Can you work these out from the model? Positions are in its coordinate system, mm. A direction names the side the tool comes from. Round coordinates to 2 decimals unless told otherwise and drop trailing zeros. Order: outer loops, then holes, each group sorted by start corner. A loop starts at its lowest first (then second) coordinate and runs counter-clockwise, first axis right, second up. Notation, with made-up numbers: (-10.5, 83.25) - (42.5, 83.25) arc R23 cw to (42.5, 100.25) - close; hole circle Ø7 at (-37.75, 9). An arc over 180 degrees is marked (long way). Write item = value, one per line.
from build123d import *

# Parameters (mm, degrees)
SKETCH1_R              = 5.207
BOSS_EXTRUDE1_DEPTH    = 3.175
SKETCH2_W              = 65.278
SKETCH2_H              = 25.4
BOSS_EXTRUDE2_DEPTH    = 3.175
FILLET1_R              = 3.175
CONVERT_SOLID1_DEPTH   = 65.278
CONVERT_SOLID1_2_DEPTH = 65.278


# Read off the part's stored shape, not the designer's step: Convert-Solid1
with BuildPart() as part:
    # Sketch1 → Boss-Extrude1 (new body)
    with BuildSketch(Plane.XY):
        with BuildLine():
            Line((0, 0), (65.278, 0))
            Line((65.278, 0), (65.278, 66.802))
            ThreePointArc((65.278, 66.802), (56.515, 75.565), (47.752, 66.802))
            ThreePointArc((47.752, 66.802), (32.639, 51.689), (17.526, 66.802))
            ThreePointArc((17.526, 66.802), (8.763, 75.565), (0, 66.802))
            Line((0, 66.802), (0, 0))
        make_face()
        with Locations((8.763, 66.802)):
            Circle(SKETCH1_R, mode=Mode.SUBTRACT)
        with Locations((56.515, 66.802)):
            Circle(SKETCH1_R, mode=Mode.SUBTRACT)
    extrude(amount=BOSS_EXTRUDE1_DEPTH)

    # Sketch2 → Boss-Extrude2 (add)
    with BuildSketch(Plane(origin=(0, 0, 0), x_dir=(1, 0, 0), z_dir=(0, 1, 0))):
        with Locations((32.639, -15.875)):
            Rectangle(SKETCH2_W, SKETCH2_H)
        with BuildLine():
            Line((16.764, -15.73022), (16.764, -20.81022))
            ThreePointArc((16.764, -20.81022), (12.7, -24.87422), (8.636, -20.81022))
            Line((8.636, -20.81022), (8.636, -15.73022))
            ThreePointArc((8.636, -15.73022), (12.7, -11.66622), (16.764, -15.73022))
        make_face(mode=Mode.SUBTRACT)
        with BuildLine():
            Line((48.514, -15.73022), (48.514, -20.81022))
            ThreePointArc((48.514, -20.81022), (52.578, -24.87422), (56.642, -20.81022))
            Line((56.642, -20.81022), (56.642, -15.73022))
            ThreePointArc((56.642, -15.73022), (52.578, -11.66622), (48.514, -15.73022))
        make_face(mode=Mode.SUBTRACT)
    extrude(amount=BOSS_EXTRUDE2_DEPTH)

    # Fillet1
    fillet1_edges = [part.edges().sort_by_distance(p)[0] for p in [
        (0, 1.5875, 28.575),
        (65.278, 1.5875, 28.575),
    ]]
    fillet(fillet1_edges, radius=FILLET1_R)

    # Convert-Solid1 outline → Convert-Solid1 (cut)
    with BuildSketch(Plane.YZ):
        with BuildLine():
            ThreePointArc((6.35, 0), (1.859871939, 1.859871939), (0, 6.35))
            Line((0, 6.35), (0, 0))
            Line((0, 0), (6.35, 0))
        make_face()
    extrude(amount=CONVERT_SOLID1_DEPTH, mode=Mode.SUBTRACT)

    # Convert-Solid1 2 outline → Convert-Solid1 2 (add)
    with BuildSketch(Plane.YZ):
        with BuildLine():
            ThreePointArc((6.35, 3.175), (4.10493597, 4.10493597), (3.175, 6.35))
            Line((3.175, 6.35), (3.175, 3.175))
            Line((3.175, 3.175), (6.35, 3.175))
        make_face()
    extrude(amount=CONVERT_SOLID1_2_DEPTH)


solid = part.part
(1) If we section it at B-B (x = 12.7): Write out the boundary of the cut face in (y, z) (3 decimals).
Computed:
outline = (0, 6.35) arc R6.35 ccw to (6.35, 0) - (63.394, 0) - (63.394, 3.175) - (6.35, 3.175) arc R3.175 cw to (3.175, 6.35) - (3.175, 11.666) - (0, 11.666) - close; (0, 24.874) - (3.175, 24.874) - (3.175, 28.575) - (0, 28.575) - close; (70.21, 0) - (74.631, 0) - (74.631, 3.175) - (70.21, 3.175) - close
(2) If we section it at D-D (y = 15): Write out the boundary of the cut face in (x, z) (3 decimals), plus the area to 3 significant figures.
Computed:
outline = (0, 0) - (65.278, 0) - (65.278, 3.175) - (0, 3.175) - close
area = 207 mm^2
(3) On a 3-axis mill with a long thin cutter (end or side, diameter ignored), from which of +Z, -Z, +X, -X, +Y, -Y can I reach the whole of each face in a straight line? I mean faces 1 (the face through (12.789, 1.565, 24.873)), 2 (the face through (8.085, 71.965, 1.565)), 3 (the face through (32, 3.175, 17)). Say none if no direction works.
Computed:
face_1 = +Y, -Y
face_2 = +Z, -Z
face_3 = +Z, +X, -X, +Y
(4) If I drill on line 1 (Z direction, x = 30, y = 35) (3 decimals); line 2 (Y direction, x = 5.5, z = 2), over which ranges is the centre line in solid material (lowest first)? Write a range as from..to.
Computed:
line_1 = 0..3.175
line_2 = 1.72..62.74, 70.86..74.93
(5) Thinking about a two-plate mould opening in Z: for faces 4 (the face through (52.677, 70.321, 1.565)), 5 (the face through (32, 2, 28.575)), 6 (the face through (52.667, 1.565, 11.667)), which applies, +Z half, -Z half, draft (parallel to the pull), parting line (faces both ways), or undercut?
Computed:
face_4 = draft
face_5 = +Z half
face_6 = undercut
(6) If we section it at C-C (z = 2.25): Write out the boundary of the cut face in (x, y) (3 decimals).
Computed:
outline = (0, 1.501) - (65.278, 1.501) - (65.278, 66.802) arc R8.763 ccw to (47.752, 66.802) arc R15.113 cw to (17.526, 66.802) arc R8.763 ccw to (0, 66.802) - close; hole circle Ø10.414 at (8.763, 66.802); hole circle Ø10.414 at (56.515, 66.802)
(7) If we section it at A-A (z = 18.5): Write out the boundary of the cut face in (x, y) (3 decimals), plus the area to 3 significant figures.
Computed:
outline = (0, 0) - (8.636, 0) - (8.636, 3.175) - (0, 3.175) - close; (16.764, 0) - (48.514, 0) - (48.514, 3.175) - (16.764, 3.175) - close; (56.642, 0) - (65.278, 0) - (65.278, 3.175) - (56.642, 3.175) - close
area = 156 mm^2
(8) Will these pins go through, and if not, where does the flat tip stop? P1, Ø6.5, axis at x = 39.5, z = 22.5, coming from the +Y side (3 decimals); P2, Ø13.5, axis at x = 8.763, y = 66.802, coming from the +Z side (3 decimals); P3, Ø16.5, axis at x = 56.515, y = 66.802, coming from the -Z side; P4, Ø1, axis at x = 56, y = 63.5, coming from the +Z side.
Computed:
P1 = 3.175
P2 = 3.175
P3 = 0
P4 = through
